Part model, mm, in its own coordinate system. A direction names the side the tool comes from. Coordinates: 2 decimals unless noted, no trailing zeros. Order: outer loops, then holes, each group sorted by start corner. A loop starts at its lowest first (then second) coordinate and runs counter-clockwise, first axis right, second up.
from build123d import *

# Parameters (mm, degrees)
SKETCH1_R           = 6.5
BOSS_EXTRUDE1_DEPTH = 7
SKETCH2_W           = 22
SKETCH2_H           = 5
BOSS_EXTRUDE2_DEPTH = 15
SKETCH3_R           = 1.651
CUT_EXTRUDE1_DEPTH  = 34.301651611
FILLET1_R           = 3


with BuildPart() as part:
    # Sketch1 → Boss-Extrude1 (new body)
    with BuildSketch(Plane.XY):
        Polygon((22, 10), (-22, 10), (-22, -10), (-22, -15), (22, -15), (22, -10), align=None)
        with Locations((-12.5, 0)):
            Circle(SKETCH1_R, mode=Mode.SUBTRACT)
        with Locations((12.5, 0)):
            Circle(SKETCH1_R, mode=Mode.SUBTRACT)
    extrude(amount=BOSS_EXTRUDE1_DEPTH)

    # Sketch2 → Boss-Extrude2 (add)
    with BuildSketch(Plane(origin=(0, 0, 0), x_dir=(-1, 0, 0), z_dir=(0, 0, -1))):
        with Locations((-11, -12.5)):
            Rectangle(SKETCH2_W, SKETCH2_H)
        with Locations((11, -12.5)):
            Rectangle(SKETCH2_W, SKETCH2_H)
    extrude(amount=BOSS_EXTRUDE2_DEPTH)

    # Sketch3 → Cut-Extrude1 (cut, through all)
    with BuildSketch(Plane(origin=(0, -10, 0), x_dir=(1, 0, 0), z_dir=(0, 1, 0))):
        with Locations(Location((17.5, 11, 0), (0, 0, 270))):
            Circle(SKETCH3_R)
        with Locations(Location((0, 11, 0), (0, 0, 270))):
            Circle(SKETCH3_R)
        with Locations(Location((-17.5, 11, 0), (0, 0, 270))):
            Circle(SKETCH3_R)
    extrude(amount=-CUT_EXTRUDE1_DEPTH, mode=Mode.SUBTRACT)

    # Fillet1
    fillet1_edges = [part.edges().sort_by_distance(p)[0] for p in [
        (-22, -12.5, -15),
        (22, -12.5, -15),
    ]]
    fillet(fillet1_edges, radius=FILLET1_R)


solid = part.part
Q1. Cut at A-A on y = 6. Write the cut outline in (x, z), and give its area (3 significant figures).
Results list:
outline: (-22, 0) - (-15, 0) - (-15, 7) - (-22, 7) - close; (-10, 0) - (10, 0) - (10, 7) - (-10, 7) - close; (15, 0) - (22, 0) - (22, 7) - (15, 7) - close
area: 238 mm2
Q2. Which spindle directions (+Z, -Z, +X, -X, +Y, -Y) get a long thin tool onto all of the face, cutting with end or side? Do faces 4 (the face through (-19.1, -12.5, -11.4)), 5 (the face through (0, 0, 0)). Say none if no direction does.
Results list:
face 4: +Y, -Y
face 5: -Z, +X, -X, +Y
Q3. Wall check: line 1 along X through (y, z) = (-12.65, -11); line 2 along Y through (x, z) = (-12.5, 2.75); line 3 along X through (y, z) = (1.5, 5.5). Give the ranges that are in metal, low to high.
Results list:
line 1: x = -22 to -19.15, -15.85 to -1.65, 1.65 to 15.85, 19.15 to 22
line 2: y = -15 to -6.5, 6.5 to 10
line 3: x = -22 to -18.82, -6.18 to 6.18, 18.82 to 22
Q4. Cut at D-D on x = -17.5. Write the cut outline in (y, z), and give its area (3 significant figures).
Results list:
outline: (-15, -15) - (-10, -15) - (-10, -12.65) - (-15, -12.65) - close; (-15, -9.35) - (-10, -9.35) - (-10, 0) - (-4.15, 0) - (-4.15, 7) - (-15, 7) - close; (4.15, 0) - (10, 0) - (10, 7) - (4.15, 7) - close
area: 175 mm2
Q5. Cut at B-B on z = -11. Write the cut outline in (x, y).
Results list:
outline: (-22, -15) - (-19.15, -15) - (-19.15, -10) - (-22, -10) - close; (-15.85, -15) - (-1.65, -15) - (-1.65, -10) - (-15.85, -10) - close; (1.65, -15) - (15.85, -15) - (15.85, -10) - (1.65, -10) - close; (19.15, -15) - (22, -15) - (22, -10) - (19.15, -10) - close
Q6. Pin check, flat tips, straight feed: pin 1 Ø7.5 at (x, z) = (5, -6) entering from +Y; pin 2 Ø2.5 at (x, z) = (0, -11) entering from -Y; pin 3 Ø15 at (x, y) = (12.5, 0) entering from -Z. Stop position of each tip, or through.
Results list:
pin 1: stops at y = -10
pin 2: passes through
pin 3: stops at z = 0
Q7. Mould opens along Z. For faces 1 (the face through (-21.1, -12.46, -14.14)), 2 (the face through (0.496, -12.465, -9.425)), 3 (the face through (18.7, 1.95, 3.45)) say: pulls with the +Z half, pulls with the -Z half, needs draft (parallel to the pull), parting line crosses it, or undercut.
Results list:
face 1: pulls with the -Z half
face 2: undercut
face 3: needs draft
Q8. Cut at C-C on x = 12.5. Write the cut outline in (y, z).
Results list:
outline: (-15, -15) - (-10, -15) - (-10, 0) - (-6.5, 0) - (-6.5, 7) - (-15, 7) - close; (6.5, 0) - (10, 0) - (10, 7) - (6.5, 7) - close
